from build123d import *

# Parameters (mm, degrees)
SKETCH1_R           = 23.6982
SKETCH1_R_2         = 22.225
BOSS_EXTRUDE1_DEPTH = 368.3
CUT_EXTRUDE1_START  = -77.831769
SKETCH2_W           = 3.175
SKETCH2_H           = 50.546
CUT_EXTRUDE1_DEPTH  = 1.529969
CIRPATTERN2_COUNT   = 3


with BuildPart() as part:
    # Sketch1 → Boss-Extrude1 (new body)
    with BuildSketch(Plane.XY):
        Circle(SKETCH1_R)
        Circle(SKETCH1_R_2, mode=Mode.SUBTRACT)
    extrude(amount=BOSS_EXTRUDE1_DEPTH)

    # Sketch2 → Cut-Extrude1 (cut)
    with BuildSketch(Plane(origin=(0, 100, 0), x_dir=(1, 0, 0), z_dir=(0, 1, 0)).offset(CUT_EXTRUDE1_START)):
        with Locations((0, -282.956)):
            Rectangle(SKETCH2_W, SKETCH2_H)
    cut_extrude1 = extrude(amount=CUT_EXTRUDE1_DEPTH, mode=Mode.SUBTRACT)

    # CirPattern2: Cut-Extrude1 ×3 about axis
    cirpattern2_axis = Axis((0, 0, 0), (0, 0, 1))
    for i in range(1, CIRPATTERN2_COUNT):
        add(cut_extrude1.rotate(cirpattern2_axis, i * 360 / CIRPATTERN2_COUNT), mode=Mode.SUBTRACT)


solid = part.part
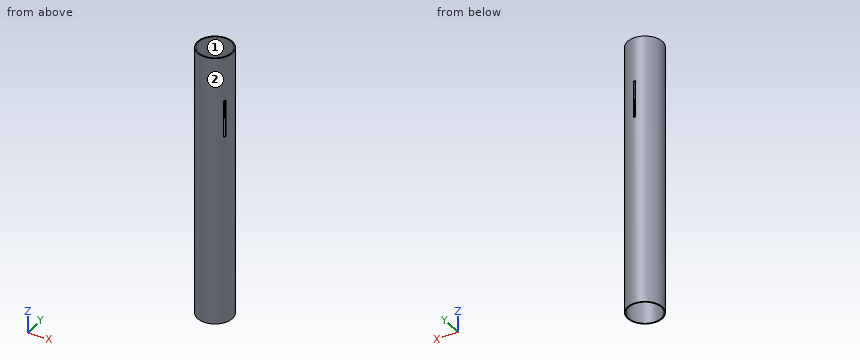
The listing builds one solid part. Answer for the finished solid, in the listing's coordinates (mm). Face numbers are marked on the shaded views. Round coordinates to 2 decimals unless told otherwise and drop trailing zeros. Write each loop counter-clockwise with the first axis right and the second up, starting at its lowest first coordinate (ties: lowest second). Pieces come first, ordered by that corner, then holes. Notation, with made-up numbers: M 88,86 L 101,86 A7 cw 101,95 Z; hole C 83.5,58 d10. An arc over 180 degrees is marked long. Write each question's results on one line, items separated by ' | '. Start each with the question number.
Item 1: Find section A-A on z = 280. Give the number of separate pieces and of enclosed holes in the cut face, and give its area (3 significant figures).
Item 2: Given pin 1 Ø8 at (y, z) = (8.5, 166.5) entering from -X; pin 2 Ø3 at (x, y) = (20.5, -12) entering from -Z; pin 3 Ø6 at (x, z) = (0.5, 42.5) entering from +Y; pin 4 Ø3 at (y, z) = (13, 98) entering from +X, each flat-ended and moving along its own axis, determine where each tip first touches the part or whether it passes through.
Item 3: Find section D-D on z = 344. Write down the section's boundary in (x, y) (3 decimals), and give its area (3 significant figures).
Item 4: Find section B-B on y = 0. Write down the section's boundary in (x, z) (3 decimals).
Item 5: Find section C-C on x = -12. Write down the section's boundary in (y, z), and give its area (3 significant figures).
Item 6: The mould has two halves that part along X. Classify the marked faces 1 and 2: +X half, -X half, draft (parallel to the pull), parting line (faces both ways), or undercut.
Item 7: Straight lines are drawn through the part: probe 1 along X at (y, z) = (0.5, 46); probe 2 along Y at (x, z) = (0, 144) (3 decimals); probe 3 along Y at (x, z) = (-10, 166.5). For each, find the intervals that lie inside material, in ascending order.
Answer block:
1) separate pieces: 3 | enclosed holes: 0 | area: 198 mm²
2) pin 1: stops at x = -23.27 | pin 2: stops at z = 0 | pin 3: stops at y = 23.7 | pin 4: stops at x = 20.72
3) outline: C 0,0 d47.396; hole C 0,0 d44.45 | area: 213 mm²
4) outline: M -23.698,0 L -22.225,0 L -22.225,368.3 L -23.698,368.3 Z; M 22.225,0 L 23.698,0 L 23.698,368.3 L 22.225,368.3 Z
5) outline: M -20.44,0 L -18.71,0 L -18.71,368.3 L -20.44,368.3 Z; M 18.71,0 L 20.44,0 L 20.44,368.3 L 18.71,368.3 Z | area: 1,270 mm²
6) face 1: undercut | face 2: parting line
7) probe 1: x = -23.69 to -22.22, 22.22 to 23.69 | probe 2: y = -23.698 to -22.225, 22.225 to 23.698 | probe 3: y = -21.48 to -19.85, 19.85 to 21.48
